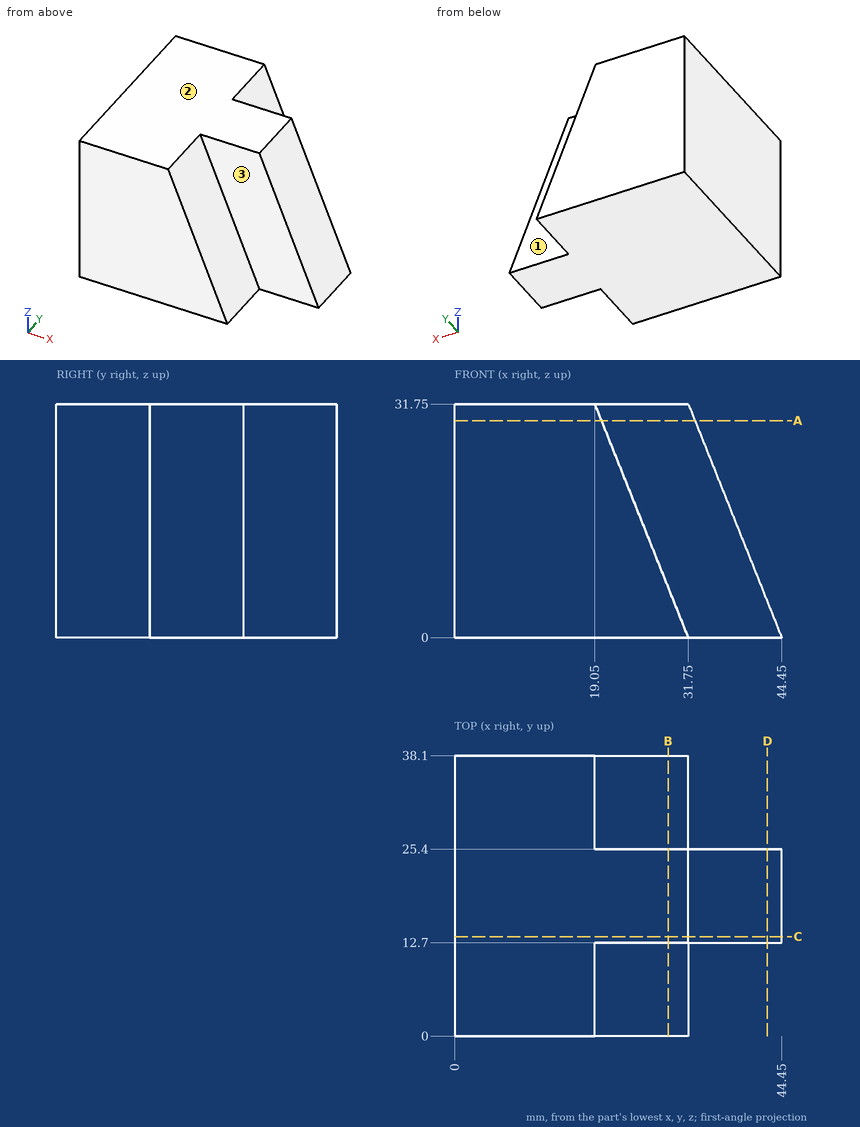
Can you work these out from the drawing? Everything is in mm from the part's minimum corner. A direction names the side the tool comes from. Give positions to 0.01 mm unless a question says otherwise; leave off trailing zeros. Order: outer loops, then holes, each group sorted by start corner. A loop starts at its lowest first (then second) coordinate and runs counter-clockwise, first axis right, second up. Notation, with made-up numbers: M -20.75,53.25 L 10.25,53.25 A19 ccw 10.25,76.25 Z; hole C -9,-4 d10. An arc over 180 degrees is marked long. Use a Markdown table: item, result. Add a question column.
1. Suppose I cut it at D-D (x = 42.5). List the corners of the cut face in (y, z) for me (3 decimals), and give its area (3 significant figures).
2. Suppose I cut it at C-C (y = 13.5). List the corners of the cut face in (x, z) for me.
3. On a 3-axis mill with a long thin cutter (end or side, diameter ignored), from which of +Z, -Z, +X, -X, +Y, -Y can I reach the whole of each face in a straight line? I mean the marked faces 1, 2 and 3. Say none if no direction works.
4. I need wall thicknesses on probe 1 along Y at (x, z) = (38.5, 10); probe 2 along X at (y, z) = (31, 29); probe 3 along X at (y, z) = (21.5, 26.5). Which ranges of each line are inside material? Lowest first, please. Write a range as from..to.
5. For pin 1 Ø5 at (x, z) = (38.5, 20) entering from -Y; pin 2 Ø6 at (y, z) = (32.5, 25) entering from +X; pin 3 Ø3 at (x, y) = (39.5, 27) entering from -Z, each with a flat end and sliding along its axis, tell me the tip position at first contact or that it passes through.
6. Suppose I cut it at B-B (x = 29). List the corners of the cut face in (y, z) for me (3 decimals), and give its area (3 significant figures).
7. Suppose I cut it at A-A (z = 29.5). List the corners of the cut face in (x, y) for me, and give its area (3 significant figures).
Results list:
| question | item | result |
|---|---|---|
| 1 | outline | M 12.7,0 L 25.4,0 L 25.4,4.875 L 12.7,4.875 Z |
| 1 | area | 61.9 mm² |
| 2 | outline | M 0,0 L 44.45,0 L 31.75,31.75 L 0,31.75 Z |
| 3 | face 1 | +Z, +X, +Y |
| 3 | face 2 | +Z, +X, -X, +Y, -Y |
| 3 | face 3 | +Z, +X, -Y |
| 4 | probe 1 | y = 12.7..25.4 |
| 4 | probe 2 | x = 0..20.15 |
| 4 | probe 3 | x = 0..33.85 |
| 5 | pin 1 | stops at y = 12.7 |
| 5 | pin 2 | stops at x = 22.95 |
| 5 | pin 3 | passes through |
| 6 | outline | M 0,0 L 38.1,0 L 38.1,6.875 L 25.4,6.875 L 25.4,31.75 L 12.7,31.75 L 12.7,6.875 L 0,6.875 Z |
| 6 | area | 578 mm² |
| 7 | outline | M 0,0 L 19.95,0 L 19.95,12.7 L 32.65,12.7 L 32.65,25.4 L 19.95,25.4 L 19.95,38.1 L 0,38.1 Z |
| 7 | area | 921 mm² |
